Part model, mm, in its own coordinate system. A direction names the side the tool comes from. Give positions to 0.01 mm unless a question says otherwise; leave off trailing zeros. Write each loop counter-clockwise with the first axis right and the second up, starting at its lowest first coordinate (ties: lowest second). Pieces come first, ordered by that corner, then holes. Notation, with made-up numbers: M 86.5,72 L 142.5,72 A16 ccw 142.5,82 Z; hole C -20,-11 d11. An arc over 180 degrees is marked long. Use CSV: the item, a comma, the result in double quotes. Start each with the question number.
Item 1: Cut at C-C (x = -42.25). List the corners of the cut face in (y, z), then the cut area to 3 significant figures.
Item 2: Drill centre lines: line 1 (Z direction, x = 42.25, y = 7); line 2 (X direction, y = 13, z = 56); line 3 (X direction, y = 24, z = 56). Where is each one in solid material? Low to high. Write a range as [from, to].
Item 3: Cut at B-B (y = 5). Count the separate pieces of the cut face and the enclosed holes in it, then the cut area to 3 significant figures.
Item 4: Cut at D-D (x = 10.25). List the corners of the cut face in (y, z).
Item 5: Which spindle directions (+Z, -Z, +X, -X, +Y, -Y) get a long thin tool onto all of the face, cutting with end or side? Do faces 5 (the flat face through (62, 16, -17.94)), 6 (the flat face through (45.4, 20, -45.8)), 7 (the flat face through (-19.078, 33, 1)). Say none if no direction does.
Item 6: Mould opens along X. For faces 1 (the cylindrical face through (27, 10, -56)), 2 (the flat face through (72.25, 17, 1)), 3 (the flat face through (-3, 33, -17.553)), 4 (the flat face through (-17, 0, -1)) say: released by +X, released by -X, zero draft, split by the parting line, or undercut.
Item 7: Cut at A-A (z = 56.19). List the corners of the cut face in (x, y).
from build123d import *

# Parameters (mm, degrees)
SKETCH1_W           = 144.5
SKETCH1_H           = 172.38
BOSS_EXTRUDE1_DEPTH = 35
CUT_EXTRUDE1_REACH  = 37
SKETCH6_R           = 10.5
SKETCH6_R_2         = 1.99
SKETCH7_W           = 32
SKETCH7_H           = 37
CUT_EXTRUDE2_DEPTH  = 5
SKETCH8_W           = 14
SKETCH8_H           = 8
CUT_EXTRUDE3_DEPTH  = 3
SKETCH9_R           = 15.25
SKETCH9_R_2         = 16
CUT_EXTRUDE4_DEPTH  = 20


with BuildPart() as part:
    # Sketch1 → Boss-Extrude1 (new body)
    with BuildSketch(Plane(origin=(0, 0, 0), x_dir=(1, 0, 0), z_dir=(0, 1, 0))):
        Rectangle(SKETCH1_W, SKETCH1_H)
    extrude(amount=BOSS_EXTRUDE1_DEPTH)

    # Sketch6 → Cut-Extrude1 (cut, up to next)
    with BuildSketch(Plane(origin=(0, 35, 0), x_dir=(1, 0, 0), z_dir=(0, 1, 0)), mode=Mode.PRIVATE) as cut_extrude1_sk1:
        with Locations((42.25, -56.19)):
            Circle(SKETCH6_R)
    cut_extrude1_tool1 = extrude(cut_extrude1_sk1.sketch, amount=-CUT_EXTRUDE1_REACH, mode=Mode.PRIVATE) & part.part
    add(cut_extrude1_tool1.solids().sort_by_distance((42.25, 35, 56.19))[0], mode=Mode.SUBTRACT)
    # Sketch6 → Cut-Extrude1 (cut, up to next)
    with BuildSketch(Plane(origin=(0, 35, 0), x_dir=(1, 0, 0), z_dir=(0, 1, 0)), mode=Mode.PRIVATE) as cut_extrude1_sk2:
        with Locations((-10.25, -56.19)):
            Circle(SKETCH6_R_2)
    cut_extrude1_tool2 = extrude(cut_extrude1_sk2.sketch, amount=-CUT_EXTRUDE1_REACH, mode=Mode.PRIVATE) & part.part
    add(cut_extrude1_tool2.solids().sort_by_distance((-10.25, 35, 56.19))[0], mode=Mode.SUBTRACT)
    # Sketch6 → Cut-Extrude1 (cut, up to next)
    with BuildSketch(Plane(origin=(0, 35, 0), x_dir=(1, 0, 0), z_dir=(0, 1, 0)), mode=Mode.PRIVATE) as cut_extrude1_sk3:
        with Locations((-42.25, -56.19)):
            Circle(SKETCH6_R)
    cut_extrude1_tool3 = extrude(cut_extrude1_sk3.sketch, amount=-CUT_EXTRUDE1_REACH, mode=Mode.PRIVATE) & part.part
    add(cut_extrude1_tool3.solids().sort_by_distance((-42.25, 35, 56.19))[0], mode=Mode.SUBTRACT)
    # Sketch6 → Cut-Extrude1 (cut, up to next)
    with BuildSketch(Plane(origin=(0, 35, 0), x_dir=(1, 0, 0), z_dir=(0, 1, 0)), mode=Mode.PRIVATE) as cut_extrude1_sk4:
        with Locations((42.25, 56.19)):
            Circle(SKETCH6_R)
    cut_extrude1_tool4 = extrude(cut_extrude1_sk4.sketch, amount=-CUT_EXTRUDE1_REACH, mode=Mode.PRIVATE) & part.part
    add(cut_extrude1_tool4.solids().sort_by_distance((42.25, 35, -56.19))[0], mode=Mode.SUBTRACT)
    # Sketch6 → Cut-Extrude1 (cut, up to next)
    with BuildSketch(Plane(origin=(0, 35, 0), x_dir=(1, 0, 0), z_dir=(0, 1, 0)), mode=Mode.PRIVATE) as cut_extrude1_sk5:
        with Locations((10.25, 56.19)):
            Circle(SKETCH6_R_2)
    cut_extrude1_tool5 = extrude(cut_extrude1_sk5.sketch, amount=-CUT_EXTRUDE1_REACH, mode=Mode.PRIVATE) & part.part
    add(cut_extrude1_tool5.solids().sort_by_distance((10.25, 35, -56.19))[0], mode=Mode.SUBTRACT)
    # Sketch6 → Cut-Extrude1 (cut, up to next)
    with BuildSketch(Plane(origin=(0, 35, 0), x_dir=(1, 0, 0), z_dir=(0, 1, 0)), mode=Mode.PRIVATE) as cut_extrude1_sk6:
        with Locations((-42.25, 56.19)):
            Circle(SKETCH6_R)
    cut_extrude1_tool6 = extrude(cut_extrude1_sk6.sketch, amount=-CUT_EXTRUDE1_REACH, mode=Mode.PRIVATE) & part.part
    add(cut_extrude1_tool6.solids().sort_by_distance((-42.25, 35, -56.19))[0], mode=Mode.SUBTRACT)
    # Sketch6 → Cut-Extrude1 (cut, up to next)
    with BuildSketch(Plane(origin=(0, 35, 0), x_dir=(1, 0, 0), z_dir=(0, 1, 0)), mode=Mode.PRIVATE) as cut_extrude1_sk7:
        with BuildLine():
            Line((-10.455537495, 9.828784258), (-1.333860018, 0.707106781))
            ThreePointArc((-1.333860018, 0.707106781), (0.373246763, 0), (-1.333860018, -0.707106781))
            Line((-1.333860018, -0.707106781), (-10.455537495, -9.828784258))
            ThreePointArc((-10.455537495, -9.828784258), (-10.455537495, -13.647160877), (-6.637160877, -13.647160877))
            Line((-6.637160877, -13.647160877), (7.01, 0))
            Line((7.01, 0), (-6.637160877, 13.647160877))
            ThreePointArc((-6.637160877, 13.647160877), (-10.455537495, 13.647160877), (-10.455537495, 9.828784258))
        make_face()
    cut_extrude1_tool7 = extrude(cut_extrude1_sk7.sketch, amount=-CUT_EXTRUDE1_REACH, mode=Mode.PRIVATE) & part.part
    add(cut_extrude1_tool7.solids().sort_by_distance((-0.05515, 35, 6.582011))[0], mode=Mode.SUBTRACT)
    # Sketch6 → Cut-Extrude1 (cut, up to next)
    with BuildSketch(Plane(origin=(0, 35, 0), x_dir=(1, 0, 0), z_dir=(0, 1, 0)), mode=Mode.PRIVATE) as cut_extrude1_sk8:
        Polygon((67.25, 20.94), (67.25, 17.44), (65.25, 17.44), (65.25, 17.94), (59.25, 17.94), (59.25, 17.44), (57.25, 17.44), (57.25, 17.94), (57.25, 20.94), align=None)
    cut_extrude1_tool8 = extrude(cut_extrude1_sk8.sketch, amount=-CUT_EXTRUDE1_REACH, mode=Mode.PRIVATE) & part.part
    add(cut_extrude1_tool8.solids().sort_by_distance((62.25, 35, -19.330625))[0], mode=Mode.SUBTRACT)

    # Sketch7 → Cut-Extrude2 (cut)
    with BuildSketch(Plane(origin=(0, 35, 0), x_dir=(1, 0, 0), z_dir=(0, 1, 0))):
        with Locations((-3.07777663, -0.946773822)):
            Rectangle(SKETCH7_W, SKETCH7_H)
    extrude(amount=-CUT_EXTRUDE2_DEPTH, mode=Mode.SUBTRACT)

    # Sketch8 → Cut-Extrude3 (cut)
    with BuildSketch(Plane(origin=(0, 35, 0), x_dir=(1, 0, 0), z_dir=(0, 1, 0))):
        with Locations((62.2, 19.2)):
            Rectangle(SKETCH8_W, SKETCH8_H)
    extrude(amount=-CUT_EXTRUDE3_DEPTH, mode=Mode.SUBTRACT)

    # Sketch9 → Cut-Extrude4 (cut)
    with BuildSketch(Plane.XZ):
        with Locations((42.25, -56.19)):
            Circle(SKETCH9_R)
        with Locations((-150, -137.51)):
            Circle(SKETCH9_R_2)
        with Locations((42.25, 56.19)):
            Circle(SKETCH9_R)
        with Locations((-42.25, 56.19)):
            Circle(SKETCH9_R)
    extrude(amount=-CUT_EXTRUDE4_DEPTH, mode=Mode.SUBTRACT)


solid = part.part
Worked answers:
1,outline,"M 0,-86.19 L 35,-86.19 L 35,-66.69 L 0,-66.69 Z; M 0,-45.69 L 35,-45.69 L 35,45.69 L 20,45.69 L 20,40.94 L 0,40.94 Z; M 0,71.44 L 20,71.44 L 20,66.69 L 35,66.69 L 35,86.19 L 0,86.19 Z"
1,area,"4,370 mm^2"
2,line 1,"z = [-86.19, -71.44], [-40.94, 40.94], [71.44, 86.19]"
2,line 2,"x = [-72.25, -57.5], [-27, -12.23], [-8.27, 27], [57.5, 72.25]"
2,line 3,"x = [-72.25, -52.75], [-31.75, -12.23], [-8.27, 31.75], [52.75, 72.25]"
3,separate pieces,"1"
3,enclosed holes,"8"
3,area,"22,100 mm^2"
4,outline,"M 0,-86.19 L 35,-86.19 L 35,-58.18 L 0,-58.18 Z; M 0,-54.2 L 35,-54.2 L 35,-17.55 L 30,-17.55 L 30,19.45 L 35,19.45 L 35,86.19 L 0,86.19 Z"
5,face 5,"+Y, -Y"
5,face 6,"-Y"
5,face 7,"+Y"
6,face 1,"undercut"
6,face 2,"released by +X"
6,face 3,"undercut"
6,face 4,"zero draft"
7,outline,"M -72.25,0 L -57.5,0 L -57.5,20 L -52.75,20 L -52.75,35 L -72.25,35 Z; M -31.75,20 L -27,20 L -27,0 L -12.24,0 L -12.24,35 L -31.75,35 Z; M -8.26,0 L 27,0 L 27,20 L 31.75,20 L 31.75,35 L -8.26,35 Z; M 52.75,20 L 57.5,20 L 57.5,0 L 72.25,0 L 72.25,35 L 52.75,35 Z"
